Job drawing, mm, ordinate dimensions from the low corner. One solid piece. A direction names the side the tool comes from. Give positions to 0.01 mm unless a question says otherwise; leave off trailing zeros. Order: outer loops, then holes, each group sorted by start corner. A loop starts at its lowest first (then second) coordinate and runs counter-clockwise, first axis right, second up. Notation, with made-up numbers: (33, -24) - (84, -24) arc R21 cw to (84, -20) - close; hole circle Ø7 at (76, 35.25). An arc over 180 degrees is marked (long way). Use one line per item in the form item = value. Start each with the question number.
1. Tool access for the marked faces 5 and 6: list every direction of +Z, -Z, +X, -X, +Y, -Y with a clear straight run to the whole face (end or side of a thin tool).
2. Band-saw the part on D-D, the plane y = 24.5. List the corners of the cut face in (x, z), plus the area to 3 significant figures.
3. Pin check, flat tip, straight feed: P1, Ø1.5, axis at x = 4, z = 6, coming from the +Y side. Stop position of the tip, or through.
4. Drill centre lines: line 1 (X direction, y = 2.5, z = 8.75); line 2 (X direction, y = 23.25, z = 1.75); line 3 (Y direction, x = 5, z = 14.25). Where is each one in solid material? Low to high.
5. Pull direction Y, two halves, no side cores. Call the marked faces 1, 2, 3 and 4: +Y half, -Y half, draft (parallel to the pull), parting line (faces both ways), or undercut.
6. Band-saw the part on C-C, the plane x = 9. List the corners of the cut face in (y, z), plus the area to 3 significant figures.
7. Band-saw the part on A-A, the plane y = 11. List the corners of the cut face in (x, z).
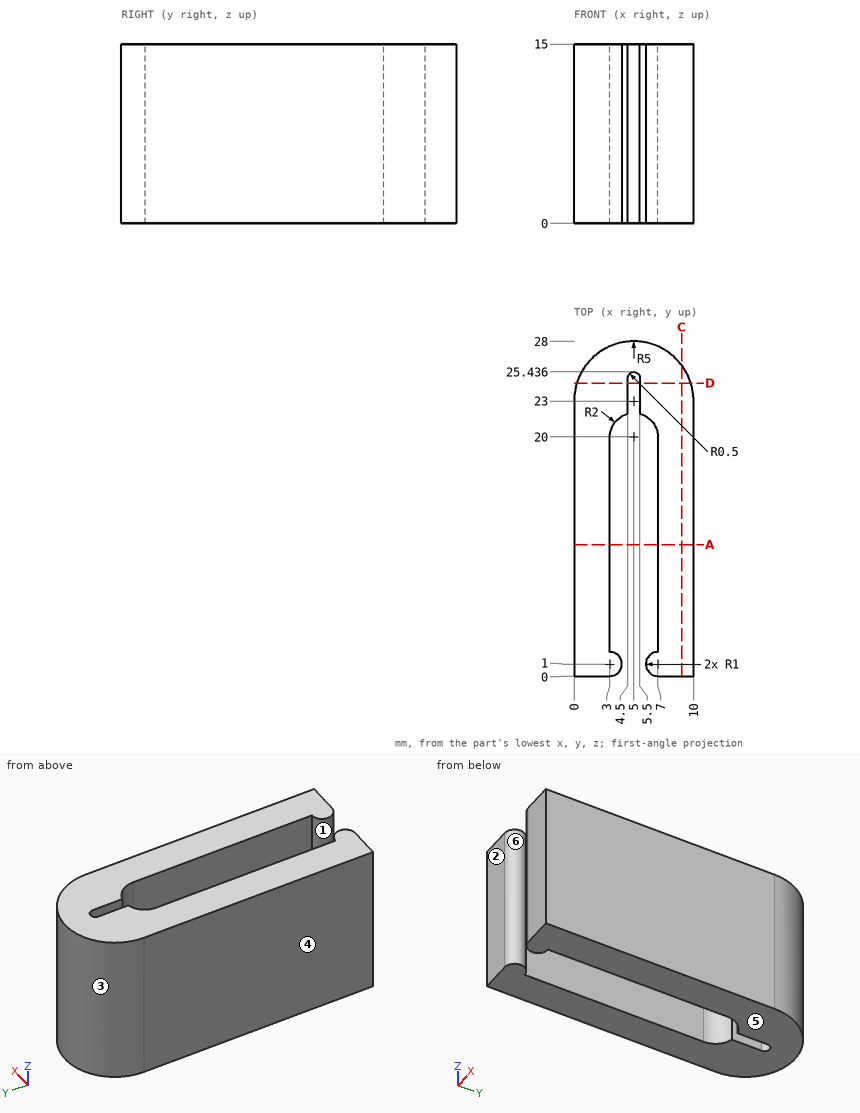
From the geometry:
q1.face_5 = -Z, +X, -X, +Y, -Y
q1.face_6 = +Z, -Z
q2.outline = (0.23, 0) - (4.5, 0) - (4.5, 15) - (0.23, 15) - close; (5.5, 0) - (9.77, 0) - (9.77, 15) - (5.5, 15) - close
q2.area = 128 mm²
q3.P1 = 27.99
q4.line_1 = 0 to 3, 7 to 10
q4.line_2 = 0.01 to 4.5, 5.5 to 9.99
q4.line_3 = 25.44 to 28
q5.face_1 = undercut
q5.face_2 = -Y half
q5.face_3 = +Y half
q5.face_4 = draft
q6.outline = (0, 0) - (26, 0) - (26, 15) - (0, 15) - close
q6.area = 390 mm²
q7.outline = (0, 0) - (3, 0) - (3, 15) - (0, 15) - close; (7, 0) - (10, 0) - (10, 15) - (7, 15) - close
